Geometry: final body of the model. Coordinates: model frame, mm. Give positions to 0.01 mm unless a question says otherwise; leave off trailing zeros. Loops run counter-clockwise (first coordinate to the right, second up) from the corner with the lowest first, then second, coordinate; pieces in that order, holes last. Notation, with made-up numbers: (36, 69.25) - (63, 69.25) arc R4 cw to (63, 73.25) - close; hole circle Ø6 at (13.25, 4). An arc over 180 degrees is marked (long way). Answer in a Markdown table with one row per item.
Autodesk Inventor part; units mm, degrees
ref_plane "YZ Plane" through (0, 0, 0) normal (1, 0, 0) x (0, 1, 0)
ref_plane "XZ Plane" through (0, 0, 0) normal (0, 1, 0) x (-1, 0, 0)
ref_plane "XY Plane" through (0, 0, 0) normal (0, 0, 1) x (1, 0, 0)
sketch "Sketch1" plane through (0, 0, 0) normal (0, 1, 0) x (-1, 0, 0)
  line L0 (-19.05, 6.35) -> (19.05, 6.35)
  line L1 (19.05, 6.35) -> (19.05, -6.35)
  line L2 (19.05, -6.35) -> (-19.05, -6.35)
  line L3 (-19.05, -6.35) -> (-19.05, 6.35)
  line L4 (-19.05, 6.35) -> (19.05, -6.35) construction
  line L5 (19.05, 6.35) -> (-19.05, -6.35) construction
  point P0 (0, 0)
  dimension "d0" = 38.1
  dimension "d1" = 12.7
extrude "Plate1" add sketch "Sketch1" along normal blind 12.7
sketch "Sketch2" plane through (19.05, 0, -6.35) normal (0, 0, -1) x (-1, 0, 0)
  line L0 (0, 0) -> (38.1, 0) construction
  line L1 (19.05, 0) -> (19.05, 12.7) construction
  line L2 (38.1, 12.7) -> (0, 12.7) construction
  point P0 (6.35, 6.35)
  point P1 (31.75, 6.35)
  dimension "d3" = 25.4
  dimension "d4" = 6.35
hole "Hole1" at (12.7, 6.35, -6.35) at (-12.7, 6.35, -6.35) direction (0, 0, 1) diameter 3.9624 end through all
sketch "Sketch3" plane through (0, 12.7, 0) normal (0, 1, 0) x (1, 0, 0)
  line L0 (-19.05, 6.35) -> (19.05, 6.35)
  point P0 (0, 0)
  point P1 (0, 0)
  dimension "d19" = 6.35
hole "Hole2" at (0, 12.7, 0) direction (0, -1, 0) diameter 3.9624 end through all
fillet "Corner Round1" radius 1.5875 4 edges at (-19.05, 6.35, -6.35) (-19.05, 6.35, 6.35) (19.05, 6.35, -6.35) (19.05, 6.35, 6.35)
equation "\"d10\" = Thickness"
equation "\"d2\" = Thickness"
equation "\"BendRadius\" = Thickness"
equation "\"BendReliefWidth\" = Thickness"
equation "\"BendReliefDepth\" = 0.5 * Thickness"
equation "\"CornerReliefSize\" = 4 * Thickness"
equation "\"MinimumRemnant\" = 2 * Thickness"
equation "\"TransitionRadius\" = BendRadius"
equation "\"JacobiRadiusSize\" = BendRadius"
equation "\"GapSize\" = Thickness"
properties part number "PLATE,NUTBLOCK,BACK" material "Aluminum 6061"
Q1. Material intervals for line 1 along X through (y, z) = (6.35, -2.5); line 2 along Y through (x, z) = (-12.7, 1); line 3 along Z through (x, y) = (0, 9.5), sorted ascending.
Check values:
| item | result |
|---|---|
| line 1 | -19.05 to -14.68, -10.72 to 10.72, 14.68 to 19.05 |
| line 2 | 0 to 4.37, 8.33 to 12.7 |
| line 3 | -6.35 to -1.98, 1.98 to 6.35 |
Q2. Cut plane D-D (y = 6.35). Give the number of separate pieces and of enclosed holes in the cut face, and give its area (3 significant figures).
Check values:
| item | result |
|---|---|
| separate pieces | 3 |
| enclosed holes | 1 |
| area | 369 mm² |
Q3. Cut plane C-C (x = 0). Output: boundary loops of the cut face in (y, z), and give its area (3 significant figures).
Check values:
| item | result |
|---|---|
| outline | (0, -6.35) - (12.7, -6.35) - (12.7, -1.98) - (0, -1.98) - close; (0, 1.98) - (12.7, 1.98) - (12.7, 6.35) - (0, 6.35) - close |
| area | 111 mm² |
Q4. Cut plane A-A (z = 0). Output: boundary loops of the cut face in (x, y).
Check values:
| item | result |
|---|---|
| outline | (-19.05, 0) - (-1.98, 0) - (-1.98, 12.7) - (-19.05, 12.7) - close; (1.98, 0) - (19.05, 0) - (19.05, 12.7) - (1.98, 12.7) - close; hole circle Ø3.96 at (-12.7, 6.35); hole circle Ø3.96 at (12.7, 6.35) |
Q5. Draft query along Y for faces 1 (the flat face through (0, 12.7, -3)), 2 (the cylindrical face through (18.6, 6.44, -5.87)), 3 (the cylindrical face through (-11.94, 8.18, 0.09)). Return one class per face: pulls with the +Y half, pulls with the -Y half, needs draft (parallel to the pull), parting line crosses it, or undercut.
Check values:
| item | result |
|---|---|
| face 1 | pulls with the +Y half |
| face 2 | needs draft |
| face 3 | undercut |
Q6. First-contact query: pin 1 (6.5 mm diameter, centred on x = 0, z = 0, fed in from +Y); pin 2 (3.5 mm diameter, centred on x = 12.7, y = 6.35, fed in from +Z). Flat tips, straight axial feed; report the tip coordinate or a pass-through.
Check values:
| item | result |
|---|---|
| pin 1 | y = 12.7 |
| pin 2 | through |
